Here's how the part is built. I have some questions about the finished solid (model axes, mm). A direction names the side the tool comes from. Coordinates: 2 decimals unless noted, no trailing zeros. Write each loop counter-clockwise with the first axis right and the second up, starting at its lowest first coordinate (ties: lowest second). Pieces come first, ordered by that corner, then holes.
Item 1: If we section it at A-A (x = 0): Please give me the cut outline in (y, z), then the cut area to 3 significant figures.
Item 2: I'm going to push flat-ended pins straight in: pin 1 Ø1 at (x, y) = (23, -8.5) entering from +Z; pin 2 Ø0.5 at (x, y) = (34, -4.5) entering from -Z. Where does each tip first touch, or does it pass through?
Item 3: We'd pull the mould along X, two halves only. Please class faces 1 (the face through (20.34, -5.01, -28.05)), 2 (the face through (23.4, -5, 23.3)), 3 (the face through (-34.65, -5, 0)): +X half, -X half, draft (parallel to the pull), parting line (faces both ways), or undercut.
Item 4: If we section it at B-B (z = 24): Please give me the cut outline in (x, y), then the cut area to 3 significant figures.
Item 5: If I drill on line 1 (X direction, y = -7.75, z = 0); line 2 (X direction, y = -3.75, z = 29), over which ranges is the centre line in solid material (lowest first)?
Item 6: For faces 4 (the face through (-32.607, -5.009, 5.205)), 5 (the face through (-28.05, -5.01, -20.34)), 6 (the face through (34, -5, -2.308)), which set-ups out of +Z, -Z, +X, -X, +Y, -Y let a thin tool reach every point of the face, with its end or its side?
from build123d import *

# Parameters (mm, degrees)
F1_DEPTH = 10.16


with BuildPart() as f1:
    # F0 (on Front) → F1 (new body)
    with BuildSketch(Plane.XZ):
        with BuildLine():
            ThreePointArc((32.9392262703, -2.3081968538), (32.9998003891, -1.1548048657), (33.02, 0))
            ThreePointArc((33.02, 0), (32.9998003891, 1.1548048657), (32.9392262703, 2.3081968538))
            ThreePointArc((32.9392262703, 2.3081968538), (32.6134690065, 5.1654660356), (32.0403378403, 7.9835550403))
            ThreePointArc((32.0403378403, 7.9835550403), (31.4038861681, 10.2037411543), (30.6137937319, 12.3740063578))
            ThreePointArc((30.6137937319, 12.3740063578), (29.4210354287, 14.9907663014), (28.0051179043, 17.4938209425))
            ThreePointArc((28.0051179043, 17.4938209425), (26.7137411543, 19.4086690307), (25.2916697641, 21.2285619047))
            ThreePointArc((25.2916697641, 21.2285619047), (23.3486659148, 23.3486659148), (21.2285619047, 25.2916697641))
            ThreePointArc((21.2285619047, 25.2916697641), (19.4086690307, 26.7137411543), (17.4938209425, 28.0051179043))
            ThreePointArc((17.4938209425, 28.0051179043), (14.9907663014, 29.4210354287), (12.3740063578, 30.6137937319))
            ThreePointArc((12.3740063578, 30.6137937319), (10.2037411543, 31.4038861681), (7.9835550403, 32.0403378403))
            ThreePointArc((7.9835550403, 32.0403378403), (5.1654660356, 32.6134690065), (2.3081968538, 32.9392262703))
            ThreePointArc((2.3081968538, 32.9392262703), (0, 33.02), (-2.3081968538, 32.9392262703))
            ThreePointArc((-2.3081968538, 32.9392262703), (-5.1654660356, 32.6134690065), (-7.9835550403, 32.0403378403))
            ThreePointArc((-7.9835550403, 32.0403378403), (-10.2037411543, 31.4038861681), (-12.3740063578, 30.6137937319))
            ThreePointArc((-12.3740063578, 30.6137937319), (-14.9907663014, 29.4210354287), (-17.4938209425, 28.0051179043))
            ThreePointArc((-17.4938209425, 28.0051179043), (-19.4086690307, 26.7137411543), (-21.2285619047, 25.2916697641))
            ThreePointArc((-21.2285619047, 25.2916697641), (-23.3486659148, 23.3486659148), (-25.2916697641, 21.2285619047))
            ThreePointArc((-25.2916697641, 21.2285619047), (-26.7137411543, 19.4086690307), (-28.0051179043, 17.4938209425))
            ThreePointArc((-28.0051179043, 17.4938209425), (-29.4210354287, 14.9907663014), (-30.6137937319, 12.3740063578))
            ThreePointArc((-30.6137937319, 12.3740063578), (-31.4038861681, 10.2037411543), (-32.0403378403, 7.9835550403))
            ThreePointArc((-32.0403378403, 7.9835550403), (-32.6134690065, 5.1654660356), (-32.9392262703, 2.3081968538))
            ThreePointArc((-32.9392262703, 2.3081968538), (-33.02, 0), (-32.9392262703, -2.3081968538))
            ThreePointArc((-32.9392262703, -2.3081968538), (-32.6134690065, -5.1654660356), (-32.0403378403, -7.9835550403))
            ThreePointArc((-32.0403378403, -7.9835550403), (-31.4038861681, -10.2037411543), (-30.6137937319, -12.3740063578))
            ThreePointArc((-30.6137937319, -12.3740063578), (-29.4210354287, -14.9907663014), (-28.0051179043, -17.4938209425))
            ThreePointArc((-28.0051179043, -17.4938209425), (-26.7137411543, -19.4086690307), (-25.2916697641, -21.2285619047))
            ThreePointArc((-25.2916697641, -21.2285619047), (-23.3486659148, -23.3486659148), (-21.2285619047, -25.2916697641))
            ThreePointArc((-21.2285619047, -25.2916697641), (-19.4086690307, -26.7137411543), (-17.4938209425, -28.0051179043))
            ThreePointArc((-17.4938209425, -28.0051179043), (-14.9907663014, -29.4210354287), (-12.3740063578, -30.6137937319))
            ThreePointArc((-12.3740063578, -30.6137937319), (-10.2037411543, -31.4038861681), (-7.9835550403, -32.0403378403))
            ThreePointArc((-7.9835550403, -32.0403378403), (-5.1654660356, -32.6134690065), (-2.3081968538, -32.9392262703))
            ThreePointArc((-2.3081968538, -32.9392262703), (0, -33.02), (2.3081968538, -32.9392262703))
            ThreePointArc((2.3081968538, -32.9392262703), (5.1654660356, -32.6134690065), (7.9835550403, -32.0403378403))
            ThreePointArc((7.9835550403, -32.0403378403), (10.2037411543, -31.4038861681), (12.3740063578, -30.6137937319))
            ThreePointArc((12.3740063578, -30.6137937319), (14.9907663014, -29.4210354287), (17.4938209425, -28.0051179043))
            ThreePointArc((17.4938209425, -28.0051179043), (19.4086690307, -26.7137411543), (21.2285619047, -25.2916697641))
            ThreePointArc((21.2285619047, -25.2916697641), (23.3486659148, -23.3486659148), (25.2916697641, -21.2285619047))
            ThreePointArc((25.2916697641, -21.2285619047), (26.7137411543, -19.4086690307), (28.0051179043, -17.4938209425))
            ThreePointArc((28.0051179043, -17.4938209425), (29.4210354287, -14.9907663014), (30.6137937319, -12.3740063578))
            ThreePointArc((30.6137937319, -12.3740063578), (31.4038861681, -10.2037411543), (32.0403378403, -7.9835550403))
            ThreePointArc((32.0403378403, -7.9835550403), (32.6134690065, -5.1654660356), (32.9392262703, -2.3081968538))
        make_face()
        with BuildLine():
            ThreePointArc((2.3081968538, 31.9206554332), (23.4321098934, 21.7989046042), (32.004, 0))
            ThreePointArc((32.004, 0), (-21.7989046042, -23.4321098934), (-2.3081968538, 31.9206554332))
            ThreePointArc((-2.3081968538, 31.9206554332), (0, 32.004), (2.3081968538, 31.9206554332))
        make_face(mode=Mode.SUBTRACT)
        with BuildLine():
            ThreePointArc((32.9392262703, 2.3081968538), (32.9998003891, 1.1548048657), (33.02, 0))
            ThreePointArc((33.02, 0), (32.9998003891, -1.1548048657), (32.9392262703, -2.3081968538))
            Line((32.9392262703, -2.3081968538), (34.6495732665, -2.3081968538))
            Line((34.6495732665, -2.3081968538), (34.6495732665, 2.3081968538))
            Line((34.6495732665, 2.3081968538), (32.9392262703, 2.3081968538))
        make_face()
        with BuildLine():
            ThreePointArc((30.6137937319, 12.3740063578), (31.4038861681, 10.2037411543), (32.0403378403, 7.9835550403))
            Line((32.0403378403, 7.9835550403), (33.6669744962, 8.5120813284))
            Line((33.6669744962, 8.5120813284), (32.2404303878, 12.9025326459))
            Line((32.2404303878, 12.9025326459), (30.6137937319, 12.3740063578))
        make_face()
        with BuildLine():
            Line((33.6669744962, -8.5120813284), (32.0403378403, -7.9835550403))
            ThreePointArc((32.0403378403, -7.9835550403), (31.4038861681, -10.2037411543), (30.6137937319, -12.3740063578))
            Line((30.6137937319, -12.3740063578), (32.2404303878, -12.9025326459))
            Line((32.2404303878, -12.9025326459), (33.6669744962, -8.5120813284))
        make_face()
        with BuildLine():
            ThreePointArc((25.2916697641, 21.2285619047), (26.7137411543, 19.4086690307), (28.0051179043, 17.4938209425))
            Line((28.0051179043, 17.4938209425), (29.3888176905, 18.4991376832))
            Line((29.3888176905, 18.4991376832), (26.6753695504, 22.2338786454))
            Line((26.6753695504, 22.2338786454), (25.2916697641, 21.2285619047))
        make_face()
        with BuildLine():
            Line((29.3888176905, -18.4991376832), (28.0051179043, -17.4938209425))
            ThreePointArc((28.0051179043, -17.4938209425), (26.7137411543, -19.4086690307), (25.2916697641, -21.2285619047))
            Line((25.2916697641, -21.2285619047), (26.6753695504, -22.2338786454))
            Line((26.6753695504, -22.2338786454), (29.3888176905, -18.4991376832))
        make_face()
        with BuildLine():
            ThreePointArc((17.4938209425, 28.0051179043), (19.4086690307, 26.7137411543), (21.2285619047, 25.2916697641))
            Line((21.2285619047, 25.2916697641), (22.2338786454, 26.6753695504))
            Line((22.2338786454, 26.6753695504), (18.4991376832, 29.3888176905))
            Line((18.4991376832, 29.3888176905), (17.4938209425, 28.0051179043))
        make_face()
        with BuildLine():
            Line((22.2338786454, -26.6753695504), (21.2285619047, -25.2916697641))
            ThreePointArc((21.2285619047, -25.2916697641), (19.4086690307, -26.7137411543), (17.4938209425, -28.0051179043))
            Line((17.4938209425, -28.0051179043), (18.4991376832, -29.3888176905))
            Line((18.4991376832, -29.3888176905), (22.2338786454, -26.6753695504))
        make_face()
        with BuildLine():
            ThreePointArc((7.9835550403, 32.0403378403), (10.2037411543, 31.4038861681), (12.3740063578, 30.6137937319))
            Line((12.3740063578, 30.6137937319), (12.9025326459, 32.2404303878))
            Line((12.9025326459, 32.2404303878), (8.5120813284, 33.6669744962))
            Line((8.5120813284, 33.6669744962), (7.9835550403, 32.0403378403))
        make_face()
        with BuildLine():
            Line((12.9025326459, -32.2404303878), (12.3740063578, -30.6137937319))
            ThreePointArc((12.3740063578, -30.6137937319), (10.2037411543, -31.4038861681), (7.9835550403, -32.0403378403))
            Line((7.9835550403, -32.0403378403), (8.5120813284, -33.6669744962))
            Line((8.5120813284, -33.6669744962), (12.9025326459, -32.2404303878))
        make_face()
        with BuildLine():
            ThreePointArc((-2.3081968538, 32.9392262703), (0, 33.02), (2.3081968538, 32.9392262703))
            Line((2.3081968538, 32.9392262703), (2.3081968538, 34.6495732665))
            Line((2.3081968538, 34.6495732665), (-2.3081968538, 34.6495732665))
            Line((-2.3081968538, 34.6495732665), (-2.3081968538, 32.9392262703))
        make_face()
        with BuildLine():
            Line((2.3081968538, -34.6495732665), (2.3081968538, -32.9392262703))
            ThreePointArc((2.3081968538, -32.9392262703), (0, -33.02), (-2.3081968538, -32.9392262703))
            Line((-2.3081968538, -32.9392262703), (-2.3081968538, -34.6495732665))
            Line((-2.3081968538, -34.6495732665), (2.3081968538, -34.6495732665))
        make_face()
        with BuildLine():
            ThreePointArc((-12.3740063578, 30.6137937319), (-10.2037411543, 31.4038861681), (-7.9835550403, 32.0403378403))
            Line((-7.9835550403, 32.0403378403), (-8.5120813284, 33.6669744962))
            Line((-8.5120813284, 33.6669744962), (-12.9025326459, 32.2404303878))
            Line((-12.9025326459, 32.2404303878), (-12.3740063578, 30.6137937319))
        make_face()
        with BuildLine():
            Line((-8.5120813284, -33.6669744962), (-7.9835550403, -32.0403378403))
            ThreePointArc((-7.9835550403, -32.0403378403), (-10.2037411543, -31.4038861681), (-12.3740063578, -30.6137937319))
            Line((-12.3740063578, -30.6137937319), (-12.9025326459, -32.2404303878))
            Line((-12.9025326459, -32.2404303878), (-8.5120813284, -33.6669744962))
        make_face()
        with BuildLine():
            ThreePointArc((-21.2285619047, 25.2916697641), (-19.4086690307, 26.7137411543), (-17.4938209425, 28.0051179043))
            Line((-17.4938209425, 28.0051179043), (-18.4991376832, 29.3888176905))
            Line((-18.4991376832, 29.3888176905), (-22.2338786454, 26.6753695504))
            Line((-22.2338786454, 26.6753695504), (-21.2285619047, 25.2916697641))
        make_face()
        with BuildLine():
            Line((-18.4991376832, -29.3888176905), (-17.4938209425, -28.0051179043))
            ThreePointArc((-17.4938209425, -28.0051179043), (-19.4086690307, -26.7137411543), (-21.2285619047, -25.2916697641))
            Line((-21.2285619047, -25.2916697641), (-22.2338786454, -26.6753695504))
            Line((-22.2338786454, -26.6753695504), (-18.4991376832, -29.3888176905))
        make_face()
        with BuildLine():
            ThreePointArc((-28.0051179043, 17.4938209425), (-26.7137411543, 19.4086690307), (-25.2916697641, 21.2285619047))
            Line((-25.2916697641, 21.2285619047), (-26.6753695504, 22.2338786454))
            Line((-26.6753695504, 22.2338786454), (-29.3888176905, 18.4991376832))
            Line((-29.3888176905, 18.4991376832), (-28.0051179043, 17.4938209425))
        make_face()
        with BuildLine():
            Line((-26.6753695504, -22.2338786454), (-25.2916697641, -21.2285619047))
            ThreePointArc((-25.2916697641, -21.2285619047), (-26.7137411543, -19.4086690307), (-28.0051179043, -17.4938209425))
            Line((-28.0051179043, -17.4938209425), (-29.3888176905, -18.4991376832))
            Line((-29.3888176905, -18.4991376832), (-26.6753695504, -22.2338786454))
        make_face()
        with BuildLine():
            ThreePointArc((-32.0403378403, 7.9835550403), (-31.4038861681, 10.2037411543), (-30.6137937319, 12.3740063578))
            Line((-30.6137937319, 12.3740063578), (-32.2404303878, 12.9025326459))
            Line((-32.2404303878, 12.9025326459), (-33.6669744962, 8.5120813284))
            Line((-33.6669744962, 8.5120813284), (-32.0403378403, 7.9835550403))
        make_face()
        with BuildLine():
            Line((-32.2404303878, -12.9025326459), (-30.6137937319, -12.3740063578))
            ThreePointArc((-30.6137937319, -12.3740063578), (-31.4038861681, -10.2037411543), (-32.0403378403, -7.9835550403))
            Line((-32.0403378403, -7.9835550403), (-33.6669744962, -8.5120813284))
            Line((-33.6669744962, -8.5120813284), (-32.2404303878, -12.9025326459))
        make_face()
        with BuildLine():
            ThreePointArc((-32.9392262703, -2.3081968538), (-33.02, 0), (-32.9392262703, 2.3081968538))
            Line((-32.9392262703, 2.3081968538), (-34.6495732665, 2.3081968538))
            Line((-34.6495732665, 2.3081968538), (-34.6495732665, -2.3081968538))
            Line((-34.6495732665, -2.3081968538), (-32.9392262703, -2.3081968538))
        make_face()
    extrude(amount=F1_DEPTH)


solid = f1.part
Answer list:
1. outline: (-10.16, -34.65) - (0, -34.65) - (0, -32) - (-10.16, -32) - close; (-10.16, 32) - (0, 32) - (0, 34.65) - (-10.16, 34.65) - close
1. area: 53.8 mm2
2. pin 1: stops at z = 24.17
2. pin 2: stops at z = -2.31
3. face 1: +X half
3. face 2: undercut
3. face 3: -X half
4. outline: (-22.68, -10.16) - (-21.17, -10.16) - (-21.17, 0) - (-22.68, 0) - close; (21.17, -10.16) - (22.68, -10.16) - (22.68, 0) - (21.17, 0) - close
4. area: 30.6 mm2
5. line 1: x = -34.65 to -32, 32 to 34.65
5. line 2: x = -19.03 to -18.22, -15.79 to -13.54, 13.54 to 15.79, 18.22 to 19.03
6. face 4: -X, +Y, -Y
6. face 5: -Z, -X, +Y, -Y
6. face 6: +X, +Y, -Y
